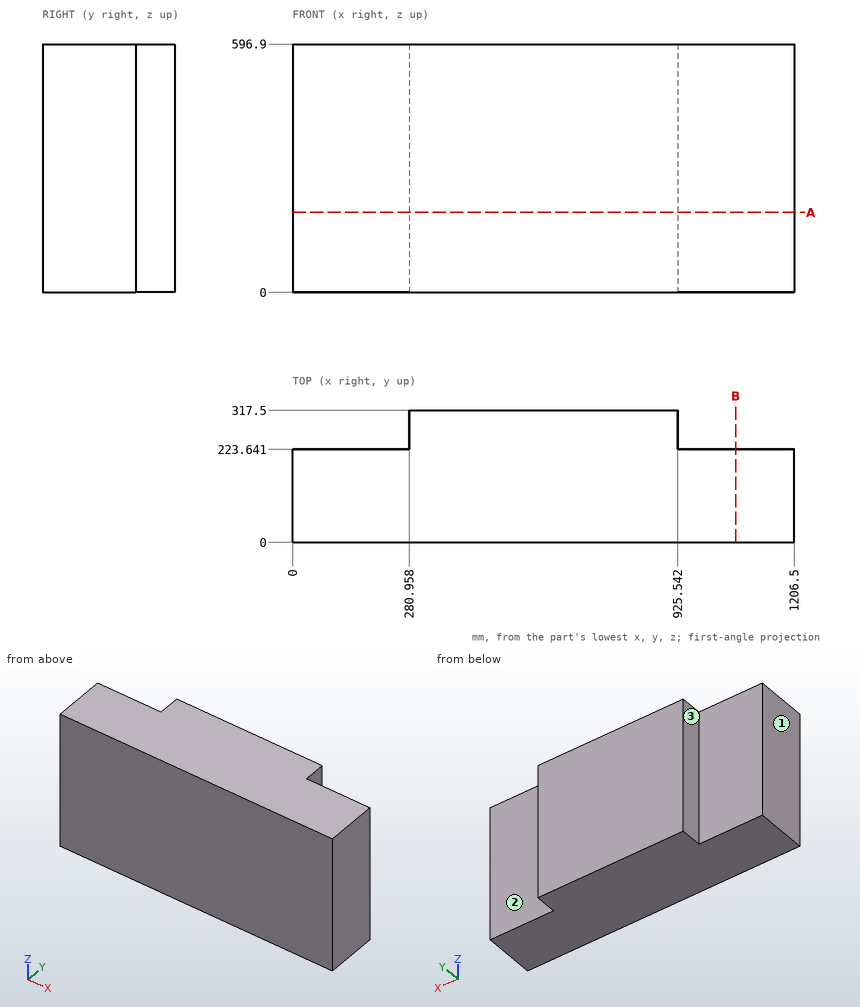
Could you check a few things on this drawing? It's one solid part, dimensions in mm from its lowest x, y, z. A direction names the side the tool comes from. Coordinates: 2 decimals unless noted, no trailing zeros. Order: outer loops, then holes, each group sorted by start corner. A loop starts at its lowest first (then second) coordinate and runs counter-clockwise, first axis right, second up. Notation, with made-up numbers: (10.5, -5.75) - (24.5, -5.75) arc R11 cw to (24.5, -1.75) - close; hole circle Ø9 at (39.5, 18.5). An arc over 180 degrees is marked (long way). One line per question, with ' | ' between items.
(1) Will this pin go through, and if not, where does the flat tip stop? pin 1 (12 mm diameter, centred on x = 531.5, y = 109, fed in from -Z).
Report:
pin 1: stops at z = 0
(2) Suppose I cut it at A-A on z = 192. List the corners of the cut face in (x, y) for me, and give its area (3 significant figures).
Report:
outline: (0, 0) - (1206.5, 0) - (1206.5, 223.64) - (925.54, 223.64) - (925.54, 317.5) - (280.96, 317.5) - (280.96, 223.64) - (0, 223.64) - close | area: 330,000 mm2
(3) If I drill on L1, parallel to Y at x = 245, z = 238.5; L2, parallel to X at y = 270, z = 361.5, over which ranges is the centre line in solid material (lowest first)?
Report:
L1: y = 0 to 223.64 | L2: x = 280.96 to 925.54
(4) Suppose I cut it at B-B on x = 1065. List the corners of the cut face in (y, z) for me.
Report:
outline: (0, 0) - (223.64, 0) - (223.64, 596.9) - (0, 596.9) - close
(5) For the marked faces 1, 2 and 3, which set-ups out of +Z, -Z, +X, -X, +Y, -Y let a thin tool reach every point of the face, with its end or its side?
Report:
face 1: +Z, -Z, -X, +Y, -Y | face 2: +Z, -Z, +X, +Y | face 3: +Z, -Z, -X, +Y
